Geometry check sheet. Reference: the model listing, model coordinates, mm. A direction names the side the tool comes from. Round coordinates to 2 decimals unless told otherwise and drop trailing zeros. Loops run counter-clockwise (first coordinate to the right, second up) from the corner with the lowest first, then second, coordinate; pieces in that order, holes last. Notation, with made-up numbers: (-11.75, 58.25) - (24.25, 58.25) arc R13 cw to (24.25, 80.25) - close; hole circle Ø6 at (78, 41.5). An arc over 180 degrees is marked (long way). Answer as CSV lines item,"result". Start each with the question number.
1) Cross-section at A-A on y = 1.5. Record the boundary of the cut face in (x, z).
2) Cross-section at C-C on x = 2. Record the boundary of the cut face in (y, z).
3) Depth check by flat-ended pin: P1, Ø2, axis at x = 0, z = 0, coming from the -Y side. Enter the tip coordinate at first touch or a pass-through.
4) Thickness scan on line 1 along Z through (x, y) = (0, 6.25); line 2 along X through (y, z) = (3.75, -0.25); line 3 along Y through (x, z) = (-0.75, 2.4). Record the ranges inside material, lowest first.
5) Cross-section at D-D on z = 1.9. Record the boundary of the cut face in (x, y).
6) Draft check along Z on faces 1 (the flat face through (2.37, 9.86, 1.394)), 2 (the flat face through (1.4, 20, -1.3)), 3 (the conical face through (-0.21, 9.12, 0.05)). Enter one of: released by +Z, released by -Z, zero draft, split by the parting line, or undercut.
7) Access from +Z, -Z, +X, -X, +Y, -Y to the whole of each face (thin tool, end or side, straight path). Record for faces 4 (the cylindrical face through (0.45, 22.96, 1.43)), 5 (the flat face through (-2.37, 9.86, -1.394)), 6 (the cylindrical face through (-1.22, 4.31, -0.27)).
8) Cross-section at B-B on y = 18.75. Record the boundary of the cut face in (x, z), and give its area (3 significant figures).
from build123d import *

# Parameters (mm, degrees)
EXTRUDE_1_DEPTH = 20
SKETCH_2_R      = 1.5
EXTRUDE_2_DEPTH = 6
M3X0_5_1_D      = 2.5
M3X0_5_1_DEPTH  = 8.5
M3X0_5_1_TIP    = 0.751075774


with BuildPart() as part:
    # ｽｹｯﾁ1 → ﾎﾞｽ - 押し出し1 (new body)
    with BuildSketch(Plane(origin=(0, 0, 0), x_dir=(1, 0, 0), z_dir=(0, 1, 0))):
        Polygon((1.58771324, -2.75), (3.175426481, 0), (1.58771324, 2.75), (-1.58771324, 2.75), (-3.175426481, 0), (-1.58771324, -2.75), align=None)
    extrude(amount=EXTRUDE_1_DEPTH)

    # ｽｹｯﾁ2 → ﾎﾞｽ - 押し出し2 (add)
    with BuildSketch(Plane(origin=(0, 20, 0), x_dir=(1, 0, 0), z_dir=(0, 1, 0))):
        with Locations(Location((0, 0, 0), (0, 0, 270))):
            Circle(SKETCH_2_R)
    extrude(amount=EXTRUDE_2_DEPTH)

    # M3x0.5 ねじ穴1
    with Locations(Plane(origin=(0, 0, 0), x_dir=(0, 0, -1), z_dir=(0, -1, 0))):
        with Locations((0, 0)):
            Hole(M3X0_5_1_D / 2, depth=M3X0_5_1_DEPTH)
            with Locations((0, 0, -(M3X0_5_1_DEPTH + M3X0_5_1_TIP / 2))):  # 118° drill point
                Cone(0, M3X0_5_1_D / 2, M3X0_5_1_TIP, mode=Mode.SUBTRACT)


solid = part.part
Answer block:
1,outline,"(-3.18, 0) - (-1.59, -2.75) - (1.59, -2.75) - (3.18, 0) - (1.59, 2.75) - (-1.59, 2.75) - close; hole circle Ø2.5 at (0, 0)"
2,outline,"(0, -2.04) - (20, -2.04) - (20, 2.04) - (0, 2.04) - close"
3,P1,"stops at y = 8.65"
4,line 1,"z = -2.75 to -1.25, 1.25 to 2.75"
4,line 2,"x = -3.03 to -1.22, 1.22 to 3.03"
4,line 3,"y = 0 to 20"
5,outline,"(-2.08, 0) - (2.08, 0) - (2.08, 20) - (-2.08, 20) - close"
6,face 1,"released by +Z"
6,face 2,"zero draft"
6,face 3,"undercut"
7,face 4,"+Y"
7,face 5,"-Z, -X, +Y, -Y"
7,face 6,"-Y"
8,outline,"(-3.18, 0) - (-1.59, -2.75) - (1.59, -2.75) - (3.18, 0) - (1.59, 2.75) - (-1.59, 2.75) - close"
8,area,"26.2 mm^2"
